from build123d import *

# Parameters (mm, degrees)
SQ_RECT_TUBING_WELDMENT_PROFILES_SQ_TUBE_DEPTH = 89.802561211
CUT_EXTRUDE1_REACH                             = 107.603


with BuildPart() as part:
    # Sketch121 → Sq_rect_tubing_weldment_profiles SQ TUBE 1 X 1 X .120 WALL(1) (new body)
    with BuildSketch(Plane(origin=(0, 0, 0), x_dir=(0.7071067811865487, 8.862608652922434e-13, -0.7071067811865464), z_dir=(0.7071067811865464, -2.139623000789053e-12, 0.7071067811865487))):
        with BuildLine():
            Line((-6.604, -12.7), (6.604, -12.7))
            ThreePointArc((6.604, -12.7), (10.914522938, -10.914522938), (12.7, -6.604))
            Line((12.7, -6.604), (12.7, 6.604))
            ThreePointArc((12.7, 6.604), (10.914522938, 10.914522938), (6.604, 12.7))
            Line((6.604, 12.7), (-6.604, 12.7))
            ThreePointArc((-6.604, 12.7), (-10.914522938, 10.914522938), (-12.7, 6.604))
            Line((-12.7, 6.604), (-12.7, -6.604))
            ThreePointArc((-12.7, -6.604), (-10.914522938, -10.914522938), (-6.604, -12.7))
        make_face()
        with BuildLine():
            Line((-6.604, -9.652), (6.604, -9.652))
            ThreePointArc((6.604, -9.652), (8.759261469, -8.759261469), (9.652, -6.604))
            Line((9.652, -6.604), (9.652, 6.604))
            ThreePointArc((9.652, 6.604), (8.759261469, 8.759261469), (6.604, 9.652))
            Line((6.604, 9.652), (-6.604, 9.652))
            ThreePointArc((-6.604, 9.652), (-8.759261469, 8.759261469), (-9.652, 6.604))
            Line((-9.652, 6.604), (-9.652, -6.604))
            ThreePointArc((-9.652, -6.604), (-8.759261469, -8.759261469), (-6.604, -9.652))
        make_face(mode=Mode.SUBTRACT)
    extrude(amount=SQ_RECT_TUBING_WELDMENT_PROFILES_SQ_TUBE_DEPTH)

    # Cut-Extrude1: up to this face of the body (flat: up to its plane)
    cut_extrude1_end = Plane(part.part.faces().sort_by_distance((31.75, -12.7, 31.75))[0])
    # Sketch122 → Cut-Extrude1 (cut, up to the picked face)
    with BuildSketch(Plane(origin=(0, 12.7, 0), x_dir=(1, 0, 0), z_dir=(8.861583310299792e-13, 1.0, 2.139725535051317e-12)), mode=Mode.PRIVATE) as cut_extrude1_sk1:
        Polygon((8.980256121, 8.980256121), (8.980256121, -26.940768363), (-8.980256121, -8.980256121), align=None)
    cut_extrude1_tool1 = split(extrude(cut_extrude1_sk1.sketch, amount=-CUT_EXTRUDE1_REACH, mode=Mode.PRIVATE), bisect_by=cut_extrude1_end, keep=Keep.BOTH, mode=Mode.PRIVATE)
    # Sketch122 → Cut-Extrude1 (cut, up to the picked face)
    with BuildSketch(Plane(origin=(0, 12.7, 0), x_dir=(1, 0, 0), z_dir=(8.861583310299792e-13, 1.0, 2.139725535051317e-12)), mode=Mode.PRIVATE) as cut_extrude1_sk2:
        Polygon((72.480256121, -54.519743879), (36.559231637, -54.519743879), (54.519743879, -72.480256121), align=None)
    cut_extrude1_tool2 = split(extrude(cut_extrude1_sk2.sketch, amount=-CUT_EXTRUDE1_REACH, mode=Mode.PRIVATE), bisect_by=cut_extrude1_end, keep=Keep.BOTH, mode=Mode.PRIVATE)
    add(cut_extrude1_tool1.solids().sort_by(Axis((2.993419, 12.7, 8.980256), (-8.861583310299792e-13, -1.0, -2.139725535051317e-12)))[0], mode=Mode.SUBTRACT)
    add(cut_extrude1_tool2.solids().sort_by(Axis((54.519744, 12.7, 60.506581), (-8.861583310299792e-13, -1.0, -2.139725535051317e-12)))[0], mode=Mode.SUBTRACT)


solid = part.part
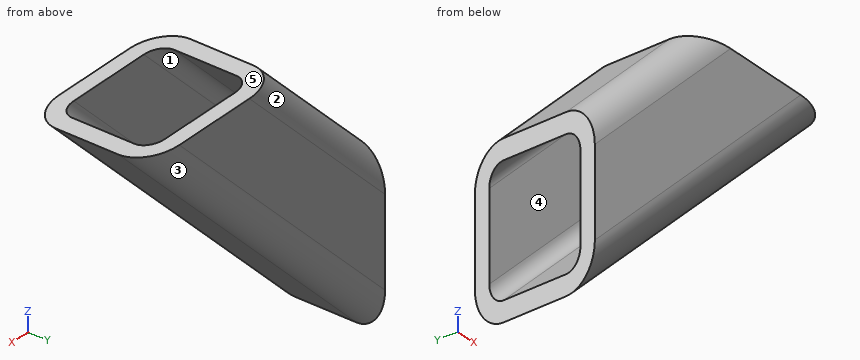
Input: part model. Units: mm. Frame: model coordinates. Face numbers are marked on the shaded views. A direction names the side the tool comes from. Give positions to 0.01 mm unless a question says otherwise; leave off trailing zeros. Write each loop counter-clockwise with the first axis right and the second up, starting at its lowest first coordinate (ties: lowest second). Pieces come first, ordered by that corner, then holes. Notation, with made-up numbers: M 4.5,12.25 L 58.5,12.25 A33 ccw 58.5,44.25 Z; hole C 23,-6 d7. An arc over 180 degrees is marked long. Write item = value, one per line. Start each with the question number.
1) Reachability of the marked faces 1 and 2 from +Z, -Z, +X, -X, +Y, -Y: full face, straight path, thin tool, end or side. Return the list, or none.
2) Cut plane B-B on y = -10.75. Return the cut outline in (x, z).
3) Draft query along Y for the marked faces 3, 4 and 5. Return one class per face: +Y half, -Y half, draft (parallel to the pull), parting line (faces both ways), or undercut.
4) Material intervals for line 1 along Z through (x, y) = (30.5, 2.5); line 2 along Y through (x, z) = (17, 12.5); line 3 along Z through (x, y) = (21.5, 5.5), sorted ascending. Write a range as [from, to].
5) First-contact query: pin 1 Ø1.5 at (x, y) = (58, -2.5) entering from +Z; pin 2 Ø8 at (x, z) = (16, 43.5) entering from -Y; pin 3 Ø4 at (x, z) = (19, -0.5) entering from -Y; pin 4 Ø1.5 at (y, z) = (0, 43.5) entering from +X. Flat tips, straight axial feed; report the tip coordinate or a pass-through.
6) Cut plane A-A on y = 1.25. Return the cut outline in (x, z), then the cut area to 3 significant figures.
Solved:
q1.face_1 = none
q1.face_2 = +Z, -X, +Y
q2.outline = M 8.98,-6.68 L 70.18,54.52 L 38.86,54.52 L 8.98,24.64 Z
q3.face_3 = +Y half
q3.face_4 = undercut
q3.face_5 = draft
q4.line_1 = [12.54, 16.85], [44.15, 48.46]
q4.line_2 = [-12.7, -9.65], [9.65, 12.7]
q4.line_3 = [3.54, 7.85], [35.15, 39.46]
q5.pin_1 = 45.1
q5.pin_2 = through
q5.pin_3 = -9.81
q5.pin_4 = 62.21
q6.outline = M 8.98,-8.98 L 72.48,54.52 L 68.17,54.52 L 8.98,-4.67 Z; M 8.98,22.63 L 40.87,54.52 L 36.56,54.52 L 8.98,26.94 Z
q6.area = 393 mm2
